Autodesk Inventor part; units mm, degrees
ref_plane "YZ Plane" through (0, 0, 0) normal (1, 0, 0) x (0, 1, 0)
ref_plane "XZ Plane" through (0, 0, 0) normal (0, 1, 0) x (-1, 0, 0)
ref_plane "XY Plane" through (0, 0, 0) normal (0, 0, 1) x (1, 0, 0)
sketch "Sketch1" plane through (0, 0, 0) normal (0, 1, 0) x (-1, 0, 0)
  line L0 (-15, 17.5) -> (15, 17.5)
  line L1 (15, 17.5) -> (15, -17.5)
  line L2 (15, -17.5) -> (-15, -17.5)
  line L3 (-15, -17.5) -> (-15, 17.5)
  line L4 (-15, 17.5) -> (15, -17.5) construction
  line L5 (15, 17.5) -> (-15, -17.5) construction
  line L6 (15, -15.5) -> (-15, -17.5)
  line L7 (21, 0) -> (-21, 0) construction
  line L8 (15, 15.5) -> (-15, 17.5)
  point P0 (0, 0)
  point P1 (0, 0)
  dimension "d1" = 30
  dimension "d2" = 35
  dimension "d19" = 31
  dimension "d20" = 30
extrude "Extrusion1" add sketch "Sketch1" against normal blind 4 contours L8 L1 L6 L3
hole "Hole1" at (0, 0, 0) direction (0, -1, 0) diameter 3.242 end through all countersink diameter 4.5 countersink angle 90
chamfer "Chamfer1" distance 0.25 angle 45 1 edges at (0, -4, -1.621)
fillet "Fillet1" radius 5 2 edges at (-15, -2, 15.5) (-15, -2, -15.5)
chamfer "Chamfer2" distance 0.5 angle 45 5 edges at (15, 0, 0) (-13.6512, -4, 14.2382) (-13.6512, -4, -14.2382) (-15, -4, 0) (15, -4, 0)
properties part number "TCSM1-002A" material "Brass, Soft Yellow"
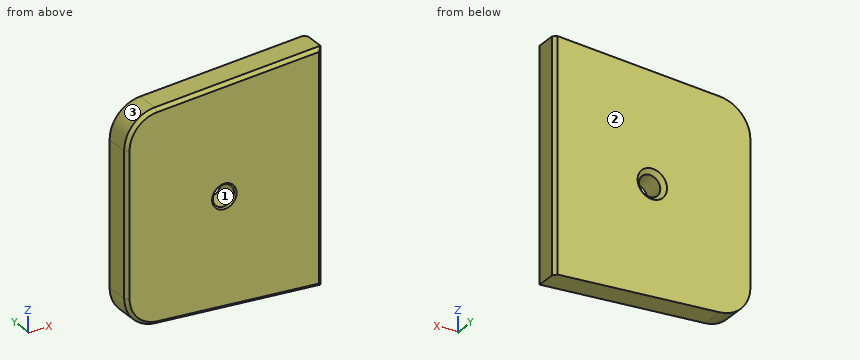
For this review, take the finished solid that the model builds, in its own axes (mm). Face numbers are marked on the shaded views. Round coordinates to 2 decimals unless told otherwise and drop trailing zeros. Loops run counter-clockwise (first coordinate to the right, second up) from the corner with the lowest first, then second, coordinate; pieces in that order, holes last.
Q1. Add section B-B on z = 0. Write out the cut boundary in (x, y).
Result sheet:
outline: (-15, -3.5) - (-14.5, -4) - (-1.87, -4) - (-1.62, -3.75) - (-1.62, -0.63) - (-2.25, 0) - (-15, 0) - close; (1.62, -3.75) - (1.87, -4) - (14.5, -4) - (15, -3.5) - (15, -0.5) - (14.5, 0) - (2.25, 0) - (1.62, -0.63) - close
Q2. Add section C-C on x = 0. Write out the cut boundary in (y, z), plus the area to 3 significant figures.
Result sheet:
outline: (-4, -16) - (-3.5, -16.5) - (0, -16.5) - (0, -2.25) - (-0.63, -1.62) - (-3.75, -1.62) - (-4, -1.87) - close; (-4, 1.87) - (-3.75, 1.62) - (-0.63, 1.62) - (0, 2.25) - (0, 16.5) - (-3.5, 16.5) - (-4, 16) - close
area: 118 mm2
Q3. To check wall thickness, follow line 1 along X through (y, z) = (-1.7, 0); line 2 along Z through (x, y) = (0, -2.25); line 3 along X through (y, z) = (-3.4, -1). State the ranges of each line that lie inside material, in increasing order.
Result sheet:
line 1: x = -15 to -1.62, 1.62 to 15
line 2: z = -16.5 to -1.62, 1.62 to 16.5
line 3: x = -15 to -1.28, 1.28 to 15
Q4. Add section A-A on y = -2.3. Write out the cut boundary in (x, z).
Result sheet:
outline: (-15, -10.82) arc R5 ccw to (-10.33, -15.81) - (15, -17.5) - (15, 17.5) - (-10.33, 15.81) arc R5 ccw to (-15, 10.82) - close; hole circle Ø3.24 at (0, 0)
Q5. Insertion check: pin 1 Ø1 at (x, y) = (-1.5, -1) entering from -Z; pin 2 Ø12 at (x, z) = (0, 0) entering from +Y; pin 3 Ø2 at (x, y) = (3, -3.5) entering from +Z. Each pin has a flat end and moves straight along its axis. Give the tip position at first contact, or say it passes through.
Result sheet:
pin 1: stops at z = -16.43
pin 2: stops at y = 0
pin 3: stops at z = 16.77
Q6. Mouldability with a two-part tool opening along Z and no side actions: class the marked faces 1, 2 and 3 as +Z half, -Z half, draft (parallel to the pull), parting line (faces both ways), or undercut.
Result sheet:
face 1: undercut
face 2: draft
face 3: +Z half
Q7. Add section D-D on x = -5.5. Write out the cut boundary in (y, z), plus the area to 3 significant figures.
Result sheet:
outline: (-4, -15.63) - (-3.5, -16.13) - (0, -16.13) - (0, 16.13) - (-3.5, 16.13) - (-4, 15.63) - close
area: 129 mm2
